The listing builds one solid part. Answer for the finished solid, in the listing's coordinates (mm). Face numbers are marked on the shaded views. A direction names the side the tool comes from. Round coordinates to 2 decimals unless told otherwise and drop trailing zeros. Order: outer loops, then holes, each group sorted by start corner. A loop starts at its lowest first (then second) coordinate and runs counter-clockwise, first axis right, second up. Notation, with made-up numbers: (30, 42.5) - (89, 42.5) arc R24 ccw to (89, 72.5) - close; hole circle Ø5 at (36.5, 11). An arc over 180 degrees is marked (long way). One line per item, written item: value. Start each with the question number.
1. Section A-A, the plane y = -22.5 is taken. Give the vertices of the cut face in (x, z).
2. Section D-D, the plane y = -19.5 is taken. Give the vertices of the cut face in (x, z), then the cut area to 3 significant figures.
3. Flat-ended cylindrical pins translate along their axes: P1, Ø12, axis at x = 28, z = 15, coming from the -Y side; P2, Ø4, axis at y = -3.5, z = 16.5, coming from the +X side; P3, Ø6, axis at y = -11.5, z = 23, coming from the +X side; P4, Ø10, axis at x = 15.5, z = 18, coming from the -Y side. Find the tip coordinate at first contact, or state that the pin passes through.
4. Section B-B, the plane x = 19 is taken. Give the vertices of the cut face in (y, z), then the cut area to 3 significant figures.
5. Section C-C, the plane z = 13.75 is taken. Give the vertices of the cut face in (x, y), then the cut area to 3 significant figures.
6. Straight lines are drawn through the part: line 1 (Z direction, x = 23.5, y = -1.25); line 2 (X direction, y = -1.5, z = 14.75); line 3 (X direction, y = -14.5, z = 13.5). For each, find the intervals that lie inside material, in ascending order.
7. A tool of negligible diameter and unlimited length cuts with its end or side. For the marked faces 1, 2, 3, 4 and 5, from which of +Z, -Z, +X, -X, +Y, -Y can it reach the whole face along a straight path? Write none if from no direction.
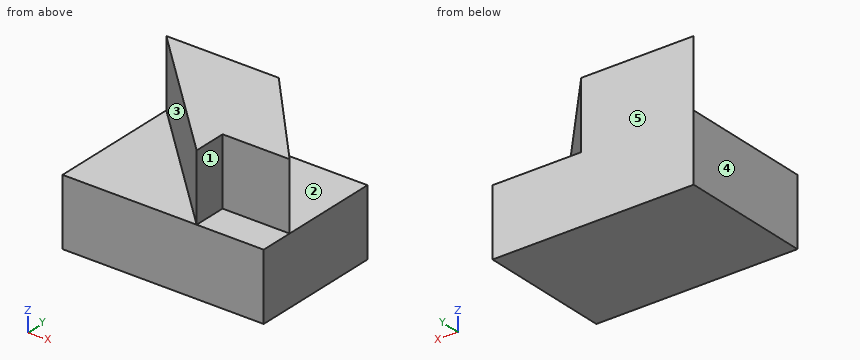
from build123d import *

# Parameters (mm, degrees)
F0_W     = 38.1
F0_H     = 25.4
F1_DEPTH = 25.4
F2_W     = 12.7
F2_H     = 12.7
F3_DEPTH = 6.35
F5_DEPTH = 12.7


with BuildPart() as f1:
    # F0 (on Front) → F1 (new body)
    with BuildSketch(Plane.XZ):
        with Locations((19.05, 12.7)):
            Rectangle(F0_W, F0_H)
    extrude(amount=F1_DEPTH)

    # F2 (on face) → F3 (cut)
    with BuildSketch(Plane.XZ.offset(25.4)):
        with Locations((31.75, 19.05)):
            Rectangle(F2_W, F2_H)
    extrude(amount=-F3_DEPTH, mode=Mode.SUBTRACT)

    # F4 (on face) → F5 (cut, symmetric)
    with BuildSketch(Plane.XY.offset(25.4)):
        Polygon((25.4, -25.4), (0, 0), (0, -25.4), align=None)
        Polygon((38.1, 0), (21.299479, 0), (38.1, -19.05), align=None)
    extrude(amount=F5_DEPTH, both=True, mode=Mode.SUBTRACT)


solid = f1.part
Answer list:
1. outline: (0, 0) - (38.1, 0) - (38.1, 12.7) - (25.4, 12.7) - (25.4, 25.4) - (22.5, 25.4) - (22.5, 12.7) - (0, 12.7) - close
2. outline: (0, 0) - (38.1, 0) - (38.1, 12.7) - (25.4, 12.7) - (25.4, 25.4) - (19.5, 25.4) - (19.5, 12.7) - (0, 12.7) - close
2. area: 559 mm²
3. P1: stops at y = -25.4
3. P2: stops at x = 26.15
3. P3: stops at x = 34.09
3. P4: stops at y = -20.5
4. outline: (-25.4, 0) - (0, 0) - (0, 25.4) - (-19, 25.4) - (-19, 12.7) - (-25.4, 12.7) - close
4. area: 564 mm²
5. outline: (0, 0) - (25.4, -25.4) - (25.4, -19.05) - (38.1, -19.05) - (21.3, 0) - close
5. area: 404 mm²
6. line 1: z = 0 to 12.7
6. line 2: x = 1.5 to 22.62
6. line 3: x = 14.5 to 34.09
7. face 1: +Z, +X, -Y
7. face 2: +Z, +X, +Y
7. face 3: +Z, -X, -Y
7. face 4: +Z, -Z, -X, +Y, -Y
7. face 5: +Z, -Z, +X, -X, +Y
